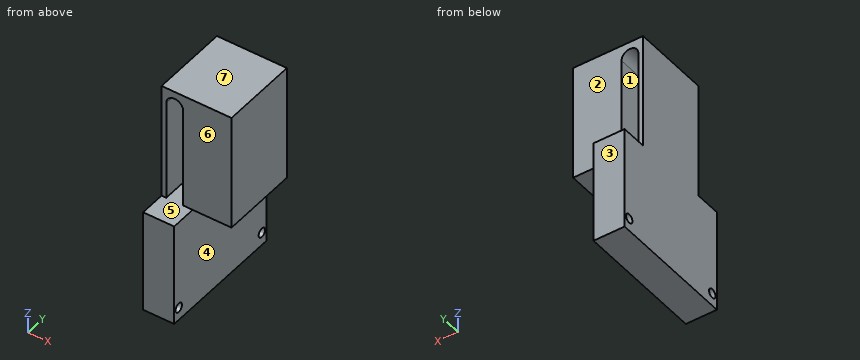
Autodesk Inventor part; units mm, degrees
ref_plane "YZ Plane" through (0, 0, 0) normal (1, 0, 0) x (0, 1, 0)
ref_plane "XZ Plane" through (0, 0, 0) normal (0, 1, 0) x (-1, 0, 0)
ref_plane "XY Plane" through (0, 0, 0) normal (0, 0, 1) x (1, 0, 0)
ref_plane "Arbeitsebene1" through (0, 0, 0) normal (0, 0, 1) x (1, 0, 0)
sketch "Skizze1" plane through (0, 0, 0) normal (0, 0, 1) x (1, 0, 0)
  circle A0 centre (-13.5, 65) radius 3 construction
  circle A1 centre (-13.5, 65) radius 3 construction
  line L0 (0, 130) -> (0, 0) construction
  line L1 (0, 130) -> (-27, 130) construction
  line L2 (-27, 0) -> (-27, 130) construction
  line L3 (0, 0) -> (-27, 0) construction
  line L4 (-27, 80) -> (0, 80)
  line L5 (0, 80) -> (0, 50)
  line L6 (0, 50) -> (-27, 50)
  line L7 (-27, 50) -> (-27, 80)
  line L8 (-27, 80) -> (0, 50) construction
  line L9 (0, 80) -> (-27, 50) construction
  dimension "d0" = 30
extrude "Extrusion1" add sketch "Skizze1" along normal blind 25
sketch "Skizze3" plane through (-27, 80, 0) normal (0, 1, 0) x (1, 0, 0)
  line L0 (0, 0) -> (0, -25)
  line L1 (0, 0) -> (5.0639, 0)
  line L2 (5.0639, 0) -> (5.0639, -24.302)
  line L3 (5.0639, -24.302) -> (0, -24.302)
  line L4 (0, -24.302) -> (0, 0)
  circle A0 centre (5.0639, -18.8642) radius 3.15
  circle A1 centre (5.0639, -8.0952) radius 3.15
  circle A2 centre (5.0639, -12.5) radius 3.25
  point P0 (27, 0)
  dimension "d6" = 6.3
  dimension "d7" = 6.3
  dimension "d10" = 6.5
extrude "Extrusion4" cut sketch "Skizze3" against normal through all contours A2 A1 L2 | L2 A1 A2 | A1 L2 A0 A2 | A2 A0 L2 | L2 A0 A2 | A1 A2 A0 L2 picked at (5.2798, -10.5577) picked at (4.848, -10.5577) picked at (5.0263, -15.7268) picked at (5.1015, -15.7268)
sketch "Skizze5" plane through (-27, 50, 0) normal (0, -1, 0) x (1, 0, 0)
  circle A0 centre (5.0639, 12.5) radius 3.25 construction
  line L0 (5.0639, 18.9193) -> (5.0639, 6.0807) construction
  line L1 (1.812, 18.9193) -> (1.812, 6.0807)
  line L2 (8.3158, 6.0807) -> (8.3158, 18.9193)
  arc A1 (8.3158, 18.9193) -> (1.812, 18.9193) centre (5.0639, 18.9193) ccw
  arc A2 (1.812, 6.0807) -> (8.3158, 6.0807) centre (5.0639, 6.0807) ccw
  point P0 (27, 0)
extrude "Extrusion6" cut sketch "Skizze5" against normal through all
sketch "Skizze6" plane through (0, 0, 0) normal (0, 0, -1) x (-1, 0, 0)
  line L0 (27, 50) -> (0, 50)
  line L1 (27, 80) -> (0, 80)
  line L2 (27, 50) -> (15, 50)
  line L3 (15, 50) -> (15, 80)
  line L4 (15, 80) -> (27, 80)
  line L5 (27, 80) -> (27, 50)
  point P0 (0, 0)
  dimension "d20" = 12
extrude "Extrusion7" add sketch "Skizze6" along normal blind 60
sketch "Skizze7" plane through (-27, 80, 25) normal (0, 1, 0) x (1, 0, 0)
  line L0 (12, 25) -> (27, 25) construction
  line L1 (12, 25) -> (12, 85) construction
  line L2 (0, 85) -> (12, 85) construction
  line L3 (0, 85) -> (0, 0) construction
  line L4 (27, 0) -> (0, 0) construction
  line L5 (27, 25) -> (27, 0) construction
  arc A0 (8.3158, 18.9193) -> (1.812, 18.9193) centre (5.0639, 18.9193) ccw construction
  line L6 (8.3158, 18.9193) -> (8.3158, 6.0807) construction
  arc A1 (1.812, 6.0807) -> (8.3158, 6.0807) centre (5.0639, 6.0807) ccw construction
  line L7 (1.812, 6.0807) -> (1.812, 18.9193) construction
  line L8 (5.0639, 18.9193) -> (5.0639, 77.8219) construction
  line L9 (8.3158, 18.9193) -> (8.3158, 77.8219)
  line L10 (1.812, 77.8219) -> (1.812, 18.9193)
  arc A2 (1.812, 18.9193) -> (8.3158, 18.9193) centre (5.0639, 18.9193) ccw
  arc A3 (8.3158, 77.8219) -> (1.812, 77.8219) centre (5.0639, 77.8219) ccw
  point P0 (27, 25)
  point P1 (5.0639, 48.3706)
extrude "Extrusion8" cut sketch "Skizze7" against normal through all
sketch "Skizze8" plane through (0, 0, 0) normal (0, 0, -1) x (-1, 0, 0)
  line L0 (15, 50) -> (15, 80)
  line L1 (15, 80) -> (0, 80)
  line L2 (0, 80) -> (0, 50)
  line L3 (0, 50) -> (15, 50)
  point P0 (0, 0)
extrude "Extrusion9" add sketch "Skizze8" along normal blind 20
sketch "Skizze10" plane through (-27, 50, 25) normal (0, -1, 0) x (1, 0, 0)
  line L0 (1.812, -77.8219) -> (1.812, -6.0807)
  arc A0 (8.3158, -6.0807) -> (1.812, -6.0807) centre (5.0639, -6.0807) ccw
  line L1 (8.3158, -6.0807) -> (8.3158, -77.8219)
  arc A1 (1.812, -77.8219) -> (8.3158, -77.8219) centre (5.0639, -77.8219) ccw
  line L2 (27, 0) -> (27, -45)
  line L3 (0, 0) -> (27, 0)
  line L4 (0, 0) -> (0, -85)
  line L5 (12, -85) -> (0, -85)
  line L6 (12, -45) -> (12, -85)
  line L7 (27, -45) -> (12, -45)
  line L8 (12, -45) -> (12, -85)
  line L9 (12, -45) -> (0, -45)
  point P0 (27, -25)
extrude "Extrusion10" add sketch "Skizze10" along normal blind 10 contours A1 L1 L9 L6 L5 L4 L0 | L0 L9 L1 A1
sketch "Skizze11" plane through (-27, 80, 25) normal (0, 1, 0) x (1, 0, 0)
  line L0 (0, 85) -> (0, 0)
  line L1 (27, 0) -> (0, 0)
  line L2 (27, 0) -> (27, 45)
  line L3 (12, 45) -> (27, 45)
  line L4 (12, 45) -> (12, 85)
  line L5 (0, 85) -> (12, 85)
  line L6 (1.812, 6.0807) -> (1.812, 77.8219)
  arc A0 (8.3158, 77.8219) -> (1.812, 77.8219) centre (5.0639, 77.8219) ccw
  line L7 (8.3158, 77.8219) -> (8.3158, 6.0807)
  arc A1 (1.812, 6.0807) -> (8.3158, 6.0807) centre (5.0639, 6.0807) ccw
  line L8 (12, 45) -> (0, 45)
  line L9 (12, 45) -> (0, 45)
  point P0 (27, 25)
extrude "Extrusion11" add sketch "Skizze11" along normal blind 10 contours L5 L4 L8 L7 A0 L6 L0 | L6 A0 L7 L8
sketch "Skizze13" plane through (-27, 40, 25) normal (0, -1, 0) x (1, 0, 0)
  line L0 (0, -85) -> (12, -85)
  line L1 (12, -85) -> (12, -45)
  line L2 (12, -45) -> (0, -45)
  line L3 (0, -45) -> (0, -85)
  point P0 (27, -25)
extrude "Extrusion12" add sketch "Skizze13" against normal up to surface (50 mm away)
sketch "Skizze14" plane through (-27, 50, 25) normal (-1, 0, 0) x (0, 0, 1)
  line L0 (-85, 40) -> (-85, -10)
  line L1 (-85, 15) -> (-0.0726, 15)
  line L2 (-85, 21.5305) -> (-80, 21.5305)
  line L3 (-80, 15) -> (-80, 37.5)
  line L4 (-80, 37.5) -> (-80, -7.5)
  circle A0 centre (-80, -7.5) radius 1.75
  circle A1 centre (-80, 37.5) radius 1.75
  point P0 (-25, -50)
  dimension "d38" = 5
  dimension "d39" = 22.5
  dimension "d40" = 45
  dimension "d41" = 3.5
  dimension "d42" = 3.5
extrude "Extrusion13" cut sketch "Skizze14" against normal through all contours A1 | A0
properties part number "kinect_fixt"
The listing builds one solid part. Answer for the finished solid, in the listing's coordinates (mm). Face numbers are marked on the shaded views. A direction names the side the tool comes from. Round coordinates to 2 decimals unless told otherwise and drop trailing zeros. Write each loop counter-clockwise with the first axis right and the second up, starting at its lowest first coordinate (ties: lowest second). Pieces come first, ordered by that corner, then holes. Notation, with made-up numbers: (-3.5, 43.5) -> (39.5, 43.5) arc R14 cw to (39.5, 59.5) -> close; hole circle Ø8 at (84.5, -10). An arc over 180 degrees is marked (long way). Use CSV: the item, a comma, the result in double quotes. Start each with the question number.
(1) Section B-B on y = 87.5 is taken. Give the vertices of the cut face in (x, z), then the cut area to 3 significant figures.
(2) Consider L1, parallel to Y at x = -22, z = -55; L2, parallel to Z at x = -22.75, y = 87.5; L3, parallel to X at y = 79, z = 15. Determine where each line is inside the solid, lowest interval first. Write a range as from..to.
(3) Section D-D on y = 78.5 is taken. Give the vertices of the cut face in (x, z), then the cut area to 3 significant figures.
(4) Section A-A on z = -55 is taken. Give the vertices of the cut face in (x, y), then the cut area to 3 significant figures.
(5) Which of the six approach directions +Z, -Z, +X, -X, +Y, -Y give full straight-line access (tool end or side, diameter ignored) to the marked faces 1, 2, 3 and 4?
(6) Section C-C on z = -13.5 is taken. Give the vertices of the cut face in (x, y).
(7) The mould has two halves that part along Z. Classify the marked faces 5, 6 and 7: released by +Z, released by -Z, zero draft, split by the parting line, or undercut.
(8) Each of these flat-tipped pins is pushed along its axis until it touches: pin 1 (8 mm diameter, centred on x = -14.5, z = 0, fed in from -Y); pin 2 (4 mm diameter, centred on y = 59, z = -37, fed in from +X); pin 3 (4 mm diameter, centred on x = -3.5, z = -21.5, fed in from +Y). Where does it stop, or does it pass through?
A:
1,outline,"(-27, -60) -> (-15, -60) -> (-15, -56.75) -> (-27, -56.75) -> close; (-27, -53.25) -> (-15, -53.25) -> (-15, -20) -> (-27, -20) -> close"
1,area,"438 mm²"
2,L1,"y = 40..40.75, 44.25..85.75, 89.25..90"
2,L2,"z = -60..-56.75, -53.25..-20"
2,L3,"x = -27..-25.19, -18.68..0"
3,outline,"(-27, -60) -> (-15, -60) -> (-15, -20) -> (0, -20) -> (0, 25) -> (-27, 25) -> close; hole (-25.19, -20) -> (-18.68, -20) -> (-18.68, 18.92) arc R3.25 ccw to (-25.19, 18.92) -> close"
3,area,"1,430 mm²"
4,outline,"(-27, 40) -> (-15, 40) -> (-15, 40.75) -> (-27, 40.75) -> close; (-27, 44.25) -> (-15, 44.25) -> (-15, 85.75) -> (-27, 85.75) -> close; (-27, 89.25) -> (-15, 89.25) -> (-15, 90) -> (-27, 90) -> close"
4,area,"516 mm²"
5,face 1,"+Y, -Y"
5,face 2,"+Z, +X, -X, +Y"
5,face 3,"+Z, -Z, +X, -X, +Y"
5,face 4,"-Z, +X, +Y, -Y"
6,outline,"(-27, 50) -> (-25.19, 50) -> (-25.19, 80) -> (-27, 80) -> close; (-18.68, 50) -> (0, 50) -> (0, 80) -> (-18.68, 80) -> close"
7,face 5,"undercut"
7,face 6,"zero draft"
7,face 7,"released by +Z"
8,pin 1,"stops at y = 50"
8,pin 2,"stops at x = -15"
8,pin 3,"stops at y = 80"
